The listing builds one solid part. Answer for the finished solid, in the listing's coordinates (mm). A direction names the side the tool comes from. Coordinates: 2 decimals unless noted, no trailing zeros. Order: outer loops, then holes, each group sorted by start corner. A loop starts at its lowest first (then second) coordinate and runs counter-clockwise, first axis right, second up. Notation, with made-up numbers: M 14,86 L 50,86 A20 cw 50,123 Z; hole C -10,9.5 d8. An arc over 180 degrees is marked long. One line per item, written item: value. Start each with the question number.
Q1. Each of these flat-tipped pins is pushed along its axis until it touches: pin 1 Ø1 at (y, z) = (14.5, -0.5) entering from +X; pin 2 Ø6 at (x, y) = (59.2, 47.25) entering from +Z; pin 3 Ø0.6 at (y, z) = (14, -0.5) entering from -X. Where does it stop, or does it pass through?
Q2. The part is cut by section D-D on x = -17.5. Give the vertices of the cut face in (y, z), then the cut area to 3 significant figures.
Q3. The part is cut by section A-A on y = -20. Give the number of separate pieces and of enclosed holes in the cut face, then the cut area to 3 significant figures.
Q4. The part is cut by section C-C on x = 6. Give the vertices of the cut face in (y, z).
Q5. Straight lines are drawn through the part: line 1 along X through (y, z) = (-30.5, 0.65); line 2 along Y through (x, z) = (-17, 0.2); line 3 along Y through (x, z) = (-35, 0.1) (3 decimals). For each, find the intervals that lie inside material, in ascending order. Write a range as [from, to].
Q6. Determine the mould class of faces 1 (the cylindrical face through (-59.815, 54.894, -0.014)), 2 (the cylindrical face through (50.752, -26.926, -0.014)), 3 (the cylindrical face through (50.972, -36.926, -0.014)), 4 (the cylindrical face through (-34, 54, 0)) for opening direction Y: pulls with the +Y half, pulls with the -Y half, needs draft (parallel to the pull), parting line crosses it, or undercut.
Q7. For faces 5 (the cylindrical face through (-34.3, 44.1, 0)), 6 (the cylindrical face through (-50.949, -27.046, -0.014)), determine the directions among +Z, -Z, +X, -X, +Y, -Y from which every point of the face is accessible in a straight line to the end or side of a thin tool.
Autodesk Inventor part; units mm, degrees
ref_plane "YZ Plane" through (0, 0, 0) normal (1, 0, 0) x (0, 1, 0)
ref_plane "XZ Plane" through (0, 0, 0) normal (0, 1, 0) x (-1, 0, 0)
ref_plane "XY Plane" through (0, 0, 0) normal (0, 0, 1) x (1, 0, 0)
sketch "Sketch1" plane through (0, 0, 0) normal (0, 0, 1) x (1, 0, 0)
  circle A0 centre (-59.5535, 47.2459) radius 7.653
  line L0 (-64.5524, 41.4512) -> (-64.5524, -23.1778)
  line L1 (-54.5526, 41.4529) -> (-54.5526, -23.5479)
  arc A1 (-54.5526, -23.5479) -> (-47.5527, -23.4962) centre (-51.0525, -23.5479) ccw
  line L2 (-47.5527, -23.4962) -> (-47.5527, 41.452)
  line L3 (-37.5474, 41.5644) -> (-37.5474, -23.5532)
  arc A2 (-64.5524, -23.1778) -> (-37.5474, -23.5515) centre (-51.0525, -23.5479) ccw
  arc A3 (-30.8632, 41.7144) -> (-37.5474, 41.5644) centre (-34.182, 40.6024) ccw
  line L4 (-30.8632, 41.7144) -> (-30.8632, -23.4297)
  line L5 (-20.7948, 41.1318) -> (-20.7948, -23.4297)
  arc A4 (-20.7947, 41.1274) -> (-47.5527, 41.452) centre (-34.182, 40.6024) ccw
  line L6 (-13.7626, 41.5703) -> (-13.7626, -23.4297)
  arc A5 (-20.7948, -23.4297) -> (-13.7626, -23.4297) centre (-17.2787, -23.4297) ccw
  line L7 (-3.7454, 41.5703) -> (-3.7454, -22.2525)
  arc A6 (-30.8632, -23.4297) -> (-3.7454, -22.2525) centre (-17.2787, -23.4297) ccw
  line L8 (3.17, 41.5703) -> (3.17, -23.406)
  line L9 (13.1831, 41.5703) -> (13.1831, -23.4297)
  arc A7 (3.17, 41.5703) -> (-3.7454, 41.5703) centre (-0.2877, 41.5703) ccw
  arc A8 (13.1831, 41.2384) -> (-13.7626, 41.5703) centre (-0.2877, 41.5703) ccw
  line L10 (20.1776, 41.5703) -> (20.1776, -23.4297)
  arc A9 (13.1831, -23.4297) -> (20.1776, -23.4297) centre (16.6804, -23.4297) ccw
  line L11 (30.1804, -22.8989) -> (30.1804, 41.5703)
  arc A10 (3.17, -23.406) -> (30.1804, -22.8989) centre (16.6804, -23.4297) ccw
  line L12 (37.1748, 41.5703) -> (37.1748, -23.4297)
  line L13 (47.1776, 41.5703) -> (47.1776, -23.4297)
  arc A11 (37.1748, 41.5703) -> (30.1804, 41.5703) centre (33.6776, 41.5703) ccw
  arc A12 (47.1776, 41.5703) -> (20.1776, 41.5703) centre (33.6776, 41.5703) ccw
  circle A13 centre (-59.5535, 47.2459) radius 3.25
  line L14 (54.172, -23.4297) -> (54.172, 41.4793)
  line L15 (64.1748, 41.4275) -> (64.1748, -23.4297)
  arc A14 (47.1776, -23.4297) -> (54.172, -23.4297) centre (50.6748, -23.4297) ccw
  arc A15 (37.1748, -23.4297) -> (64.1748, -23.4297) centre (50.6748, -23.4297) ccw
  circle A16 centre (59.2034, 47.2459) radius 7.653
  circle A17 centre (59.2034, 47.2459) radius 3.25
  point P0 (0, 0)
  point P1 (-51.0266, -27.048)
  point P2 (-51.2393, -37.0517)
extrude "Extrusion1" add sketch "Sketch1" along normal mid plane 2
properties part number "sensor2"
Output:
1. pin 1: stops at x = 64.17
1. pin 2: passes through
1. pin 3: stops at x = -64.55
2. outline: M -37.01,-1 L -26.94,-1 L -26.94,1 L -37.01,1 Z
2. area: 20.1 mm^2
3. separate pieces: 8
3. enclosed holes: 0
3. area: 160 mm^2
4. outline: M -31.7,-1 L 53.49,-1 L 53.49,1 L -31.7,1 Z
5. line 1: x = [-62.63, -39.47], [-28.88, -5.68], [5.17, 28.19], [39.17, 62.18]
5. line 2: y = [-37.01, -26.93]
5. line 3: y = [44.006, 53.975]
6. face 1: undercut
6. face 2: undercut
6. face 3: pulls with the -Y half
6. face 4: pulls with the +Y half
7. face 5: +Z, -Z, -Y
7. face 6: +Z, -Z
